Study the drawing (mm; zero at the part's minimum x, y, z) and answer. A direction names the side the tool comes from. Coordinates: 2 decimals unless noted, no trailing zeros. Order: outer loops, then holes, each group sorted by start corner. A loop starts at its lowest first (then second) coordinate and runs counter-clockwise, first axis right, second up.
1. The part is cut by section A-A, the plane z = 8. Give the vertices of the cut face in (x, y), then the cut area to 3 significant figures.
2. The part is cut by section C-C, the plane x = 0.6. Give the vertices of the cut face in (y, z).
3. The part is cut by section D-D, the plane y = 5.5. Give the vertices of the cut face in (x, z).
4. Determine the mould class of the marked faces 3, 4, 5 and 6 for opening direction Y: +Y half, -Y half, draft (parallel to the pull), parting line (faces both ways), or undercut.
5. Find the intervals of material crossed by probe 1 along Z at (x, y) = (3.2, 5.75); probe 2 along Y at (x, z) = (1.7, 18.75) (1 decimal); probe 3 along Y at (x, z) = (2.8, 5) (1 decimal), in increasing order.
6. A tool of negligible diameter and unlimited length cuts with its end or side. For the marked faces 1 and 2, from which of +Z, -Z, +X, -X, +Y, -Y can it reach the whole face along a straight path? Write none if from no direction.
7. Flat-ended cylindrical pins translate along their axes: pin 1 Ø2.5 at (x, y) = (2.75, 3.18) entering from +Z (1 decimal); pin 2 Ø1 at (y, z) = (1, 16) entering from -X. Find the tip coordinate at first contact, or state that the pin passes through.
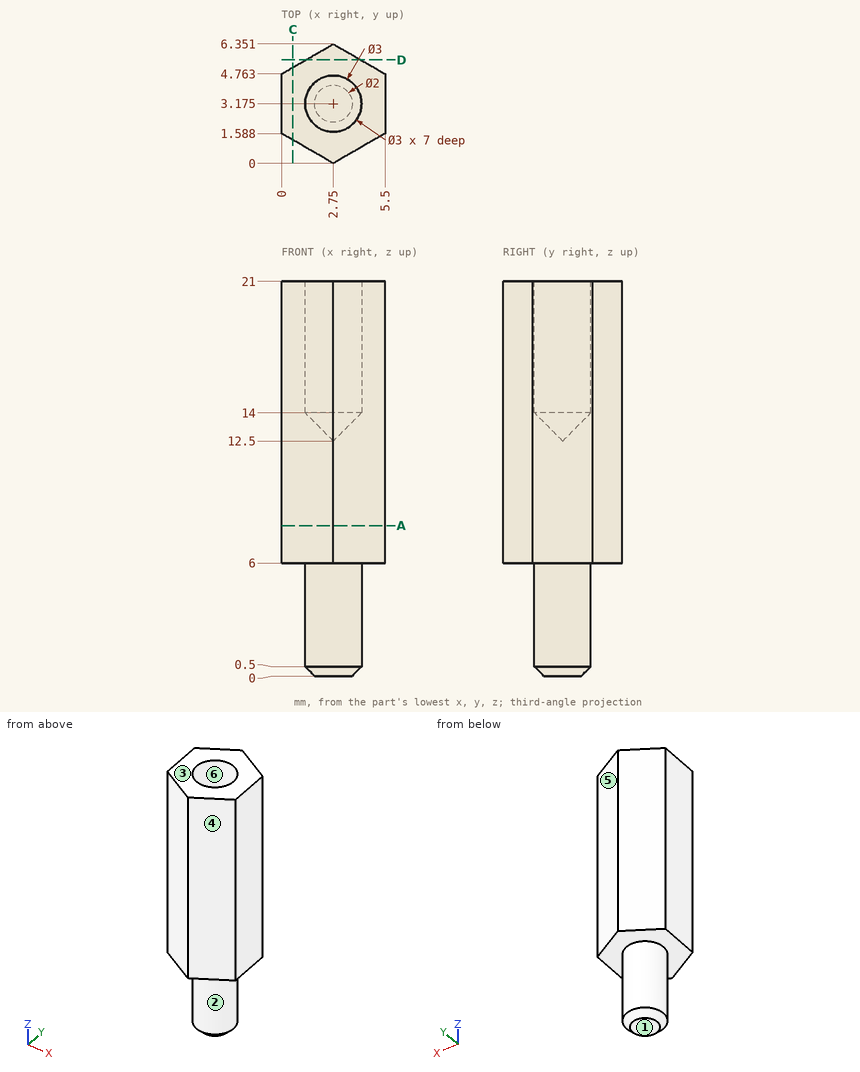
Geometry says:
1. outline: (0, 1.59) - (2.75, 0) - (5.5, 1.59) - (5.5, 4.76) - (2.75, 6.35) - (0, 4.76) - close
1. area: 26.2 mm2
2. outline: (1.24, 6) - (5.11, 6) - (5.11, 21) - (1.24, 21) - close
3. outline: (1.28, 6) - (4.22, 6) - (4.22, 21) - (1.28, 21) - close
4. face 3: draft
4. face 4: -Y half
4. face 5: +Y half
4. face 6: undercut
5. probe 1: z = 6 to 21
5. probe 2: y = 0.6 to 2.1, 4.2 to 5.7
5. probe 3: y = 1.7 to 4.7
6. face 1: -Z, +X, -X, +Y, -Y
6. face 2: -Z
7. pin 1: stops at z = 13.8
7. pin 2: stops at x = 0.15
